Verification items for the finished model (mm, model axes). Face numbers are marked on the shaded views. A direction names the side the tool comes from. Round coordinates to 2 decimals unless told otherwise and drop trailing zeros. Write each loop counter-clockwise with the first axis right and the second up, starting at its lowest first coordinate (ties: lowest second). Pieces come first, ordered by that corner, then holes. Notation, with made-up numbers: M 38,83.25 L 94,83.25 A31 cw 94,107.25 Z; hole C 49,11.25 d7. An arc over 180 degrees is marked long. Answer in a Markdown table with one row per item. Add a question column.
1. Sectioned sample at A-A on y = -7. Record the cut outline in (x, z), plus the area to 3 significant figures.
2. Sectioned sample at B-B on x = 0. Record the cut outline in (y, z), plus the area to 3 significant figures.
3. Sectioned sample at D-D on y = 16.5. Record the cut outline in (x, z), plus the area to 3 significant figures.
4. Set-up check for the marked faces 4, 5 and 6: record each of +Z, -Z, +X, -X, +Y, -Y from which the full face is reachable in a straight line by a thin tool's end or side.
5. Sectioned sample at C-C on z = 3. Record the cut outline in (x, y), plus the area to 3 significant figures.
6. Go/stop test with flat-tipped pins: pin 1 Ø3 at (y, z) = (2, 1) entering from +X; pin 2 Ø1.4 at (x, y) = (1, -6.5) entering from +Z; pin 3 Ø1.4 at (x, y) = (1, -6.5) entering from -Z. Record where each tip stops, or that it passes through.
7. Draft check along Y on the marked faces 1, 2 and 3. Enter one of: pulls with the +Y half, pulls with the -Y half, needs draft (parallel to the pull), parting line crosses it, or undercut.
8. Material ranges on probe 1 along Y at (x, z) = (4.5, -2); probe 2 along Y at (x, z) = (1, 0.25); probe 3 along Z at (x, y) = (-0.25, 18.5), recorded low to high.
```python
from build123d import *

# Parameters (mm, degrees)
SKETCH1_R           = 4
BOSS_EXTRUDE1_DEPTH = 25
SKETCH2_R           = 6
SKETCH2_R_2         = 4
BOSS_EXTRUDE2_DEPTH = 3
SKETCH3_R           = 6
BOSS_EXTRUDE3_DEPTH = 7


with BuildPart() as part:
    # Sketch1 → Boss-Extrude1 (new body)
    with BuildSketch(Plane(origin=(0, 0, 0), x_dir=(1, 0, 0), z_dir=(0, 1, 0))):
        Circle(SKETCH1_R)
    extrude(amount=BOSS_EXTRUDE1_DEPTH)

    # Sketch2 → Boss-Extrude2 (add)
    with BuildSketch(Plane.XZ):
        Circle(SKETCH2_R)
        Circle(SKETCH2_R_2, mode=Mode.SUBTRACT)
        Circle(SKETCH2_R_2)
        Circle(SKETCH2_R_2)
    extrude(amount=BOSS_EXTRUDE2_DEPTH)

    # Sketch3 → Boss-Extrude3 (add)
    with BuildSketch(Plane.XZ.offset(3)):
        Circle(SKETCH3_R)
        Polygon((4.618802154, 0), (2.309401077, 4), (-2.309401077, 4), (-4.618802154, 0), (-2.309401077, -4), (2.309401077, -4), align=None, mode=Mode.SUBTRACT)
    extrude(amount=BOSS_EXTRUDE3_DEPTH)


solid = part.part
```
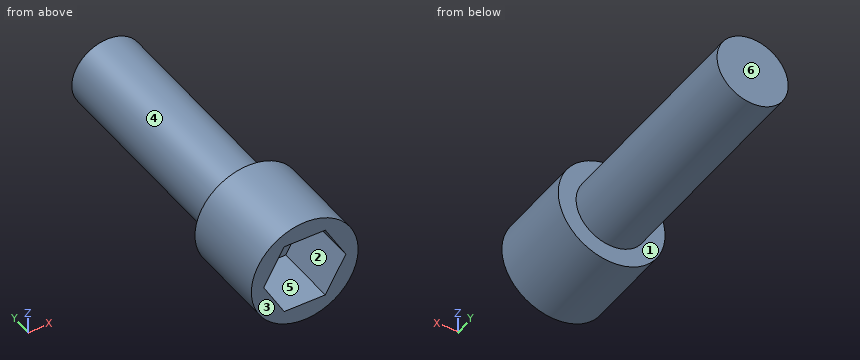
Geometry check:
| question | item | result |
|---|---|---|
| 1 | outline | C 0,0 d12; hole M -4.62,0 L -2.31,-4 L 2.31,-4 L 4.62,0 L 2.31,4 L -2.31,4 Z |
| 1 | area | 57.7 mm2 |
| 2 | outline | M -10,-6 L 0,-6 L 0,-4 L 25,-4 L 25,4 L 0,4 L 0,6 L -10,6 L -10,4 L -3,4 L -3,-4 L -10,-4 Z |
| 2 | area | 264 mm2 |
| 3 | outline | C 0,0 d8 |
| 3 | area | 50.3 mm2 |
| 4 | face 4 | +Y |
| 4 | face 5 | -Y |
| 4 | face 6 | +Z, -Z, +X, -X, +Y |
| 5 | outline | M -5.2,-10 L -2.89,-10 L -2.89,-3 L 2.89,-3 L 2.89,-10 L 5.2,-10 L 5.2,0 L 2.65,0 L 2.65,25 L -2.65,25 L -2.65,0 L -5.2,0 Z |
| 5 | area | 196 mm2 |
| 6 | pin 1 | stops at x = 4 |
| 6 | pin 2 | stops at z = 5.99 |
| 6 | pin 3 | stops at z = -5.99 |
| 7 | face 1 | pulls with the +Y half |
| 7 | face 2 | needs draft |
| 7 | face 3 | pulls with the -Y half |
| 8 | probe 1 | y = -10 to 0 |
| 8 | probe 2 | y = -3 to 25 |
| 8 | probe 3 | z = -3.99 to 3.99 |
